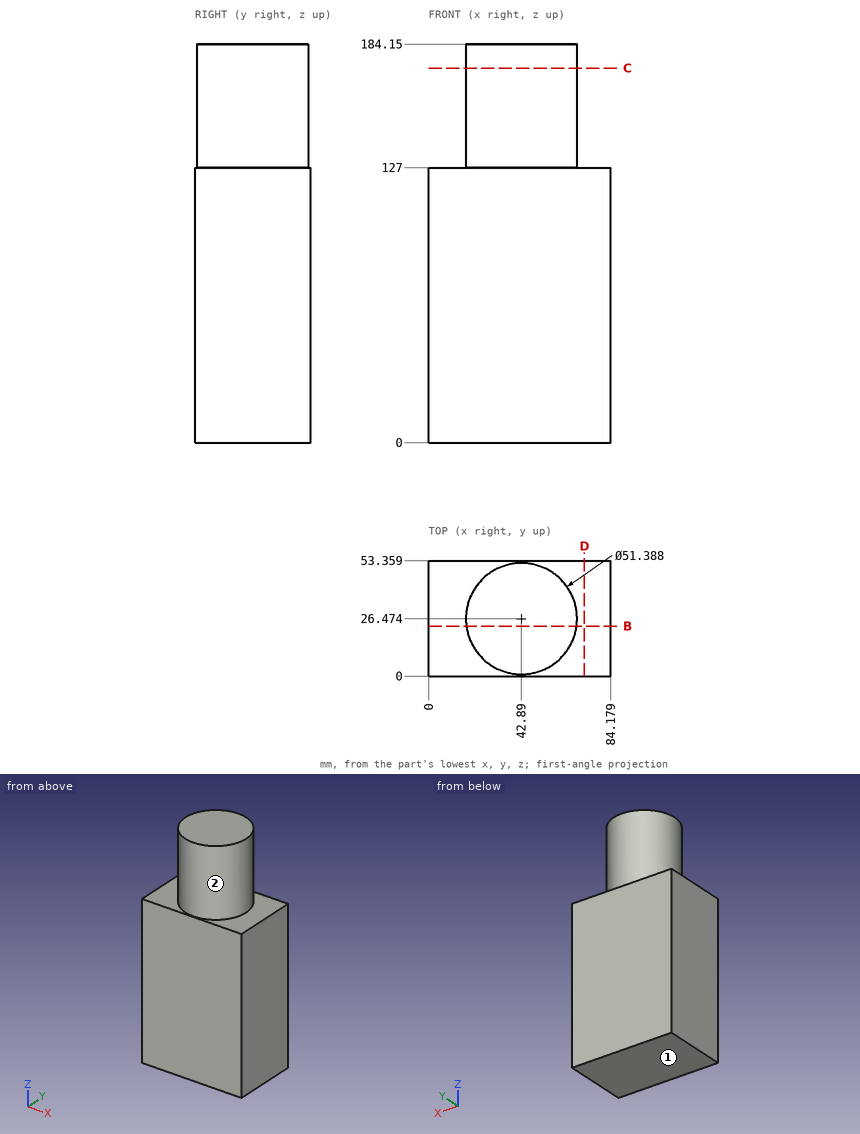
Drawing for the job (mm, zero at the part's lowest x, y, z). A direction names the side the tool comes from. Round coordinates to 2 decimals unless told otherwise and drop trailing zeros. Write each loop counter-clockwise with the first axis right and the second up, starting at its lowest first coordinate (ties: lowest second). Pieces come first, ordered by that corner, then holes. Notation, with made-up numbers: (40.5, 26) - (56.5, 26) arc R11 ccw to (56.5, 33) - close; hole circle Ø5 at (22.5, -27.75). An arc over 180 degrees is marked (long way). Write item = value, one per line. Start each with the question number.
Q1. Which spindle directions (+Z, -Z, +X, -X, +Y, -Y) get a long thin tool onto all of the face, cutting with end or side? Do the marked faces 1 and 2. Say none if no direction does.
Q2. Band-saw the part on D-D (x = 72). Give the cut face in (y, z).
Q3. Band-saw the part on C-C (z = 173). Give the cut face in (x, y), then the cut area to 3 significant figures.
Q4. Drop a flat-ended pin along its axis: pin 1 (4 mm diameter, centred on x = 68.5, z = 132, fed in from -Y) (1 decimal). Give the stop position or say it passes through.
Q5. Probe L1, parallel to Z at x = 9, y = 14.5; L2, parallel to Y at x = 65, z = 128.5 (1 decimal); L3, parallel to Y at x = 25.5, z = 139. List the from-to ranges inside material, lowest first. Write a range as from..to.
Q6. Band-saw the part on B-B (y = 23). Give the cut face in (x, z), then the cut area to 3 significant figures.
Answers below:
q1.face_1 = -Z, +X, -X, +Y, -Y
q1.face_2 = +Z
q2.outline = (0, 0) - (53.36, 0) - (53.36, 127) - (0, 127) - close
q3.outline = circle Ø51.39 at (42.89, 26.47)
q3.area = 2,070 mm2
q4.pin_1 = 16.3
q5.L1 = 0..127
q5.L2 = 13.4..39.6
q5.L3 = 7.56..45.39
q6.outline = (0, 0) - (84.18, 0) - (84.18, 127) - (68.35, 127) - (68.35, 184.15) - (17.43, 184.15) - (17.43, 127) - (0, 127) - close
q6.area = 13,600 mm2
